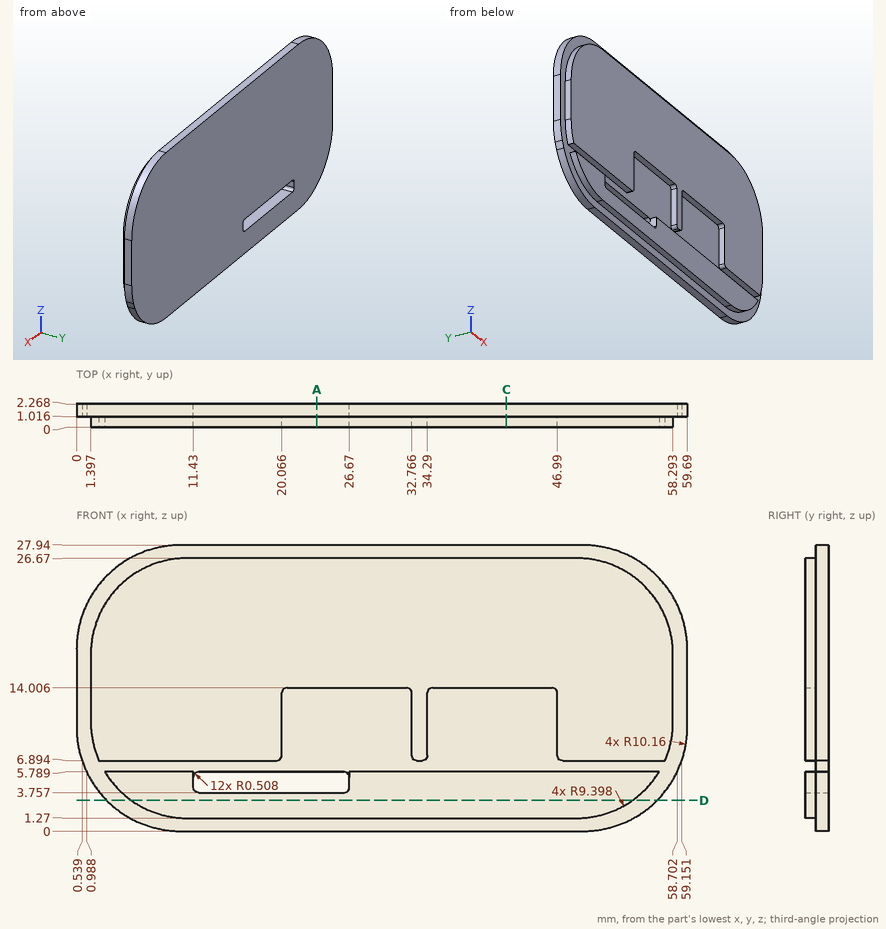
Answer from the drawing. Dimensions are ordinates in mm from the lowest x, y and z of the part. Give positions to 0.01 mm unless a question says otherwise; leave off trailing zeros. Loops run counter-clockwise (first coordinate to the right, second up) from the corner with the lowest first, then second, coordinate; pieces in that order, holes last. Notation, with made-up numbers: (29.5, 78.5) -> (74.5, 78.5) arc R33 cw to (74.5, 110.5) -> close; hole circle Ø7 at (40.5, 87). An arc over 180 degrees is marked (long way). One line per question, with ' | ' between items. Start each with the question number.
1) Section A-A, the plane x = 23.5 is taken. Determine the outline of the cut face in (y, z) (1 decimal).
2) Section C-C, the plane x = 42 is taken. Determine the outline of the cut face in (y, z) (1 decimal).
3) Section D-D, the plane z = 3 is taken. Determine the outline of the cut face in (x, y).
4) Each of these flat-tipped pins is pushed along its axis until it touches: pin 1 (0.8 mm diameter, centred on y = 0.5, z = 10, fed in from -X); pin 2 (0.5 mm diameter, centred on x = 42, y = 0.5, fed in from -Z); pin 3 (0.5 mm diameter, centred on x = 35, y = 0.5, fed in from +Z). Where does it stop, or does it pass through?
5) Straight lines are drawn through the part: L1, parallel to X at y = 0.5, z = 11.5; L2, parallel to Z at x = 38.5, y = 0.4 (1 decimal); L3, parallel to Z at x = 25, y = 1.05. For each, find the intervals that lie inside material, in ascending order.
Resolved:
1) outline: (0, 1.3) -> (1, 1.3) -> (1, 0) -> (2.3, 0) -> (2.3, 3.8) -> (0, 3.8) -> close; (0, 14) -> (1, 14) -> (1, 5.8) -> (2.3, 5.8) -> (2.3, 27.9) -> (1, 27.9) -> (1, 26.7) -> (0, 26.7) -> close
2) outline: (0, 1.3) -> (1, 1.3) -> (1, 0) -> (2.3, 0) -> (2.3, 27.9) -> (1, 27.9) -> (1, 26.7) -> (0, 26.7) -> (0, 14) -> (1, 14) -> (1, 5.8) -> (0, 5.8) -> close
3) outline: (2.95, 1.02) -> (5.36, 1.02) -> (5.36, 0) -> (54.33, 0) -> (54.33, 1.02) -> (56.74, 1.02) -> (56.74, 2.27) -> (2.95, 2.27) -> close
4) pin 1: x = 1.4 | pin 2: z = 1.27 | pin 3: z = 26.67
5) L1: 1.4 to 20.07, 32.77 to 34.29, 46.99 to 58.29 | L2: 1.3 to 5.8, 14 to 26.7 | L3: 0 to 3.76, 5.79 to 27.94
